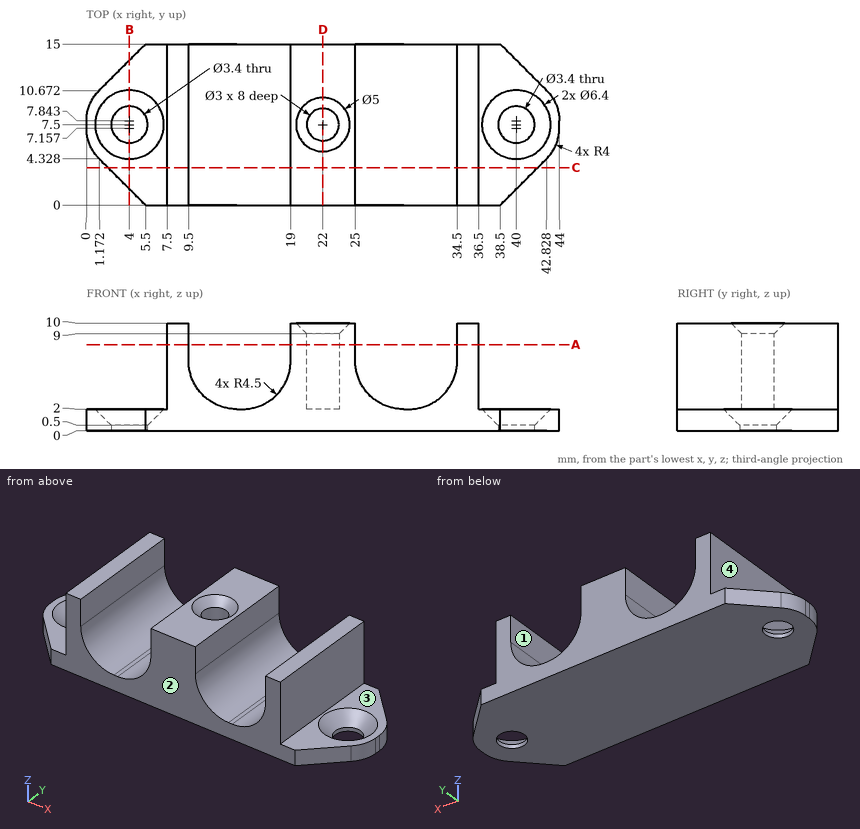
Geometry: see drawing. Coordinates: mm, zero at the bounding-box minimum. A direction names the side the tool comes from. Round coordinates to 2 decimals unless told otherwise and drop trailing zeros. Order: outer loops, then holes, each group sorted by start corner. A loop starts at its lowest first (then second) coordinate and runs counter-clockwise, first axis right, second up. Notation, with made-up numbers: (-8.5, -9.75) -> (1.5, -9.75) arc R30 ccw to (1.5, 12.25) -> close; hole circle Ø8 at (55.25, 87.25). An arc over 180 degrees is marked (long way). Answer as CSV lines item,"result".
Item 1: Section D-D, the plane x = 22. Return loops of the section in (y, z).
A:
outline,"(0, 0) -> (15, 0) -> (15, 10) -> (10, 10) -> (9, 9) -> (9, 2) -> (6, 2) -> (6, 9) -> (5, 10) -> (0, 10) -> close"
Item 2: Section B-B, the plane x = 4. Return loops of the section in (y, z).
A:
outline,"(1.5, 0) -> (5.8, 0) -> (5.8, 0.5) -> (4.3, 2) -> (1.5, 2) -> close; (9.2, 0) -> (13.5, 0) -> (13.5, 2) -> (10.7, 2) -> (9.2, 0.5) -> close"
Item 3: Section A-A, the plane z = 8. Return loops of the section in (x, y).
A:
outline,"(7.5, 0) -> (9.5, 0) -> (9.5, 15) -> (7.5, 15) -> close; (19, 0) -> (25, 0) -> (25, 15) -> (19, 15) -> close; (34.5, 0) -> (36.5, 0) -> (36.5, 15) -> (34.5, 15) -> close; hole circle Ø3 at (22, 7.5)"
Item 4: Reachability of the marked faces 1, 2, 3 and 4 from +Z, -Z, +X, -X, +Y, -Y: full face, straight path, thin tool, end or side. Return the list, or none.
A:
face 1,"+Z, +Y, -Y"
face 2,"+Z, -Z, +X, -X, -Y"
face 3,"+Z, +X, +Y, -Y"
face 4,"+Z, -X, +Y, -Y"
Item 5: Pin query (flat end, axial travel): pin 1 Ø5 at (y, z) = (4, 7) entering from +X; pin 2 Ø1.5 at (y, z) = (8, 8) entering from -X; pin 3 Ø4 at (x, y) = (39, 4.5) entering from +Z; pin 4 Ø6 at (x, z) = (6, 4.5) entering from +Y. Return the tip coordinate at first contact, or that it passes through.
A:
pin 1,"x = 36.5"
pin 2,"x = 7.5"
pin 3,"z = 2"
pin 4,"y = 15"
Item 6: Line query: L1, parallel to X at y = 1.5, z = 7.75; L2, parallel to Y at x = 22, z = 5; L3, parallel to X at y = 10.5, z = 5.5. Output: solid intervals per line, ascending.
A:
L1,"7.5 to 9.5, 19 to 25, 34.5 to 36.5"
L2,"0 to 6, 9 to 15"
L3,"7.5 to 9.61, 18.89 to 25.11, 34.39 to 36.5"
Item 7: Section C-C, the plane y = 3.5. Return loops of the section in (x, z).
A:
outline,"(2, 0) -> (42, 0) -> (42, 2) -> (36.5, 2) -> (36.5, 10) -> (34.5, 10) -> (34.5, 6.5) arc R4.5 cw to (30, 2) -> (29.5, 2) arc R4.5 cw to (25, 6.5) -> (25, 10) -> (19, 10) -> (19, 6.5) arc R4.5 cw to (14.5, 2) -> (14, 2) arc R4.5 cw to (9.5, 6.5) -> (9.5, 10) -> (7.5, 10) -> (7.5, 2) -> (2, 2) -> close"
